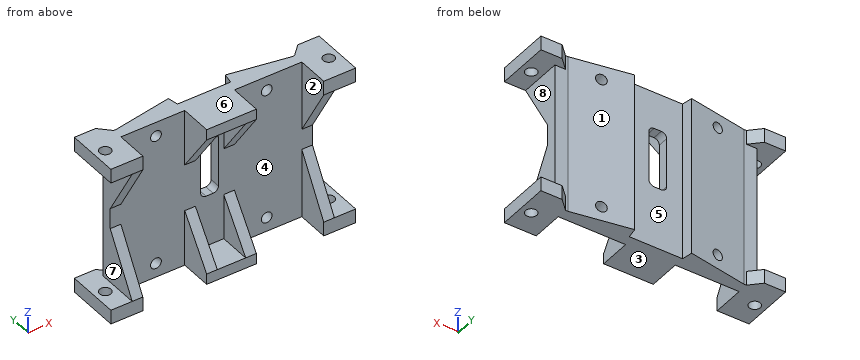
```python
from build123d import *

# Parameters (mm, degrees)
SKETCH_1_W                 = 57
SKETCH_1_H                 = 45
EXTRUDE_1_DEPTH            = 3
SKETCH_2_W                 = 4
SKETCH_2_H                 = 15
EXTRUDE_2_DEPTH            = 6
SKETCH_3_W                 = 4
SKETCH_3_H                 = 15
EXTRUDE_3_DEPTH            = 6
EXTRUDE_4_DEPTH            = 3
SKETCH_5_W                 = 4
SKETCH_5_H                 = 9
EXTRUDE_5_DEPTH            = 3
CHAMFER_1_SIZE             = 3
SKETCH_6_R                 = 1.6
CUT_EXTRUDE_1_DEPTH        = 4
SKETCH_8_W                 = 8
SKETCH_8_H                 = 3
EXTRUDE_6_DEPTH            = 9
EXTRUDE_7_DEPTH            = 3
EXTRUDE_8_DEPTH            = 3
SKETCH_12_W                = 5
SKETCH_12_H                = 17
CUT_EXTRUDE_4_DEPTH        = 3
FILLET_1_R                 = 1.5
EXTRUDE_9_REACH            = 80.57
SKETCH_15_W                = 45
SKETCH_15_H                = 17.726539555
SKETCH_16_R                = 1.5
CUT_EXTRUDE_5_DEPTH        = 79.570276896
CHAMFER_1_OF_MIRROR_2_SIZE = 3


with BuildPart() as part:
    # 草图1 → 凸台-拉伸1 (new body)
    with BuildSketch(Plane(origin=(0, 0, 0), x_dir=(1, 0, 0), z_dir=(0, 1, 0))):
        with Locations((28.5, 22.5)):
            Rectangle(SKETCH_1_W, SKETCH_1_H)
    extrude(amount=EXTRUDE_1_DEPTH)

    # 草图2 → 凸台-拉伸2 (add)
    with BuildSketch(Plane.ZY):
        with Locations((-2, -1.5)):
            Rectangle(SKETCH_2_W, SKETCH_2_H)
    extrude_2 = extrude(amount=EXTRUDE_2_DEPTH)

    # 草图3 → 凸台-拉伸3 (add)
    with BuildSketch(Plane(origin=(57, 0, 0), x_dir=(0, 0, -1), z_dir=(1, 0, 0))):
        with Locations((2, -1.5)):
            Rectangle(SKETCH_3_W, SKETCH_3_H)
    extrude_3 = extrude(amount=EXTRUDE_3_DEPTH)

    # 草图4 → 凸台-拉伸4 (add)
    with BuildSketch(Plane.ZY.offset(-57)):
        Polygon((-4, -9), (-19.588457268, 0), (0, 0), (0, -9), align=None)
    extrude_4 = extrude(amount=EXTRUDE_4_DEPTH)

    # 草图5 → 凸台-拉伸5 (add)
    with BuildSketch(Plane(origin=(0, 0, 0), x_dir=(0, 0, -1), z_dir=(1, 0, 0))):
        Polygon((19.588457268, 0), (4, 0), (4, -9), align=None)
        with Locations((2, -4.5)):
            Rectangle(SKETCH_5_W, SKETCH_5_H)
    extrude_5 = extrude(amount=EXTRUDE_5_DEPTH)

    # 倒角1
    chamfer_1_edges = [part.edges().sort_by_distance(p)[0] for p in [
        (0, 3, -2),
        (57, 3, -2),
    ]]
    chamfer(chamfer_1_edges, length=CHAMFER_1_SIZE - 0.0001)  # a hair under: the kernel refuses the full size

    # 草图6 → 切除-拉伸1 (cut)
    with BuildSketch(Plane(origin=(0, 0, -4), x_dir=(-1, 0, 0), z_dir=(0, 0, -1))):
        with Locations(Location((3, -2.323268139, 0), (0, 0, 90))):
            Circle(SKETCH_6_R)
        with Locations(Location((-60, -2.323268139, 0), (0, 0, 90))):
            Circle(SKETCH_6_R)
    cut_extrude_1 = extrude(amount=-CUT_EXTRUDE_1_DEPTH, mode=Mode.SUBTRACT)

    # 草图8 → 凸台-拉伸6 (add)
    with BuildSketch(Plane.XZ):
        with Locations((28, -43.5)):
            Rectangle(SKETCH_8_W, SKETCH_8_H)
    extrude_6 = extrude(amount=EXTRUDE_6_DEPTH)

    # 草图9 → 凸台-拉伸7 (add)
    with BuildSketch(Plane(origin=(32, 0, 0), x_dir=(0, 0, -1), z_dir=(1, 0, 0))):
        Polygon((45, 0), (29.146667939, 0), (42, -9), (45, -9), align=None)
    extrude_7 = extrude(amount=EXTRUDE_7_DEPTH)

    # 草图10 → 凸台-拉伸8 (add)
    with BuildSketch(Plane.ZY.offset(-24)):
        Polygon((-45, 0), (-45, -9), (-42, -9), (-29.146667939, 0), align=None)
    extrude_8 = extrude(amount=EXTRUDE_8_DEPTH)

    # 草图12 → 切除-拉伸4 (cut)
    with BuildSketch(Plane(origin=(0, 3, 0), x_dir=(1, 0, 0), z_dir=(0, 1, 0))):
        with Locations((28, 19)):
            Rectangle(SKETCH_12_W, SKETCH_12_H)
    extrude(amount=-CUT_EXTRUDE_4_DEPTH, mode=Mode.SUBTRACT)

    # 圆角1
    fillet_1_edges = [part.edges().sort_by_distance(p)[0] for p in [
        (25.5, 1.5, -27.5),
        (30.5, 1.5, -27.5),
        (30.5, 1.5, -10.5),
        (25.5, 1.5, -10.5),
    ]]
    fillet(fillet_1_edges, radius=FILLET_1_R)

    # 草图15 → 凸台-拉伸9 (add, up to next)
    with BuildSketch(Plane(origin=(2.119507574, 12.02032477, 0), x_dir=(0, 0, 1), z_dir=(0.17364817766693066, 0.9848077530122081, 0)), mode=Mode.PRIVATE) as extrude_9_sk1:
        with Locations((-22.5, 43.795404353)):
            Rectangle(SKETCH_15_W, SKETCH_15_H)
    extrude_9_tool1 = extrude(extrude_9_sk1.sketch, amount=-EXTRUDE_9_REACH, mode=Mode.PRIVATE) - part.part
    extrude_9 = extrude_9_tool1.solids().sort_by_distance((45.249561, 4.415333, -22.5))[0]
    add(extrude_9)

    # 草图16 → 切除-拉伸5 (cut, through all)
    with BuildSketch(Plane(origin=(2.119507574, 12.02032477, 0), x_dir=(0.9848077530122081, -0.17364817766693064, 0), z_dir=(0.17364817766693064, 0.9848077530122081, 0))):
        with Locations(Location((43.439057305, 41, 0), (0, 0, 180))):
            Circle(SKETCH_16_R)
        with Locations((43.439057305, 4)):
            Circle(SKETCH_16_R)
    cut_extrude_5 = extrude(amount=-CUT_EXTRUDE_5_DEPTH, mode=Mode.SUBTRACT)

    # 镜向1: 凸台-拉伸9, 切除-拉伸5 across plane
    add(extrude_9.mirror(Plane(origin=(28.5, 0, 0), x_dir=(0, 0, 1), z_dir=(1, 0, 0))))
    add(cut_extrude_5.mirror(Plane(origin=(28.5, 0, 0), x_dir=(0, 0, 1), z_dir=(1, 0, 0))), mode=Mode.SUBTRACT)

    # 镜向2: 凸台-拉伸2, 凸台-拉伸3, 凸台-拉伸4, 凸台-拉伸5, 切除-拉伸1 across plane
    add(extrude_2.mirror(Plane.XY.offset(-22.5)))
    add(extrude_3.mirror(Plane.XY.offset(-22.5)))
    add(extrude_4.mirror(Plane.XY.offset(-22.5)))
    add(extrude_5.mirror(Plane.XY.offset(-22.5)))
    add(cut_extrude_1.mirror(Plane.XY.offset(-22.5)), mode=Mode.SUBTRACT)

    # 倒角1 of 镜向2
    chamfer_1_of_mirror_2_edges = [part.edges().sort_by_distance(p)[0] for p in [
        (0, 3, -43),
        (57, 3, -43),
    ]]
    chamfer(chamfer_1_of_mirror_2_edges, length=CHAMFER_1_OF_MIRROR_2_SIZE - 0.0001)  # a hair under: the kernel refuses the full size

    # 镜向3: 凸台-拉伸6, 凸台-拉伸7, 凸台-拉伸8 across plane
    add(extrude_6.mirror(Plane.XY.offset(-22.5)))
    add(extrude_7.mirror(Plane.XY.offset(-22.5)))
    add(extrude_8.mirror(Plane.XY.offset(-22.5)))


solid = part.part
```
The model under review builds one solid part; all positions refer to its coordinate system, in mm. Face numbers are marked on the shaded views. A direction names the side the tool comes from. Round coordinates to 2 decimals unless told otherwise and drop trailing zeros. Loops run counter-clockwise (first coordinate to the right, second up) from the corner with the lowest first, then second, coordinate; pieces in that order, holes last.
Item 1: Take a section at A-A (z = -24). Write out the cut boundary in (x, y).
Determined:
outline: (0, 0) - (25.5, 0) - (25.5, 3) - (21, 3) - (20.48, 5.95) - (3.72, 3) - (0, 3) - close; (30.5, 0) - (57, 0) - (57, 3) - (53.28, 3) - (36.52, 5.95) - (36, 3) - (30.5, 3) - close
Item 2: Take a section at C-C (y = -7). Give the number of separate pieces and of enclosed holes in the cut face, then the cut area to 3 significant figures.
Determined:
separate pieces: 6
enclosed holes: 0
area: 304 mm2
Item 3: Take a section at D-D (z = -18.5). Write out the cut boundary in (x, y).
Determined:
outline: (0, -0.63) - (3, -0.63) - (3, 0) - (25.5, 0) - (25.5, 3) - (21, 3) - (20.48, 5.95) - (3.72, 3) - (0, 3) - close; (30.5, 0) - (54, 0) - (54, -0.63) - (57, -0.63) - (57, 3) - (53.28, 3) - (36.52, 5.95) - (36, 3) - (30.5, 3) - close
Item 4: Mouldability with a two-part tool opening along Z and no side actions: class the marked faces 5, 6, 7 and 8 as released by +Z, released by -Z, zero draft, split by the parting line, or undercut.
Determined:
face 5: zero draft
face 6: released by +Z
face 7: undercut
face 8: undercut
Item 5: For line 1 (X direction, y = -3.25, z = -6); line 2 (X direction, y = 1.25, z = -14); line 3 (Z direction, x = 30.5, y = -7.25), list the stretches that pass through material, from the lowest coordinate up.
Determined:
line 1: x = 0 to 3, 21 to 24, 32 to 35, 54 to 57
line 2: x = 0 to 25.5, 30.5 to 57
line 3: z = -45 to -42, -3 to 0
Item 6: For the marked faces 1, 2, 3 and 4, list the 3-axis set-ups (+Z, -Z, +X, -X, +Y, -Y) from which the entire face can be reached by the end or side of a thin tool; tool diameter is ignored.
Determined:
face 1: +Z, -Z, +Y
face 2: +Z, -Z, -Y
face 3: -Z, +X, -X, +Y, -Y
face 4: -Y
Item 7: Take a section at B-B (x = -3). Write out the cut boundary in (y, z).
Determined:
outline: (-9, -45) - (-3.92, -45) - (-3.92, -41) - (-9, -41) - close; (-9, -4) - (-3.92, -4) - (-3.92, 0) - (-9, 0) - close; (-0.72, -45) - (6, -45) - (6, -41) - (-0.72, -41) - close; (-0.72, -4) - (6, -4) - (6, 0) - (-0.72, 0) - close
Item 8: Clearance check with flat-ended pins moving along their axes: pin 1 Ø9 at (x, y) = (29, -4.5) entering from +Z; pin 2 Ø7 at (y, z) = (-4.5, -8) entering from +X; pin 3 Ø2.5 at (y, z) = (-6, -38.5) entering from -X; pin 4 Ø4.5 at (x, z) = (29, -27) entering from +Y. State where each tip first meets the part, or that it passes through.
Determined:
pin 1: stops at z = 0
pin 2: stops at x = 57
pin 3: stops at x = 0
pin 4: stops at y = 3
